Can you work these out from the model? Positions are in its coordinate system, mm. Face numbers are marked on the shaded views. A direction names the side the tool comes from. Round coordinates to 2 decimals unless told otherwise and drop trailing zeros. Order: outer loops, then holes, each group sorted by start corner. A loop starts at its lowest first (then second) coordinate and runs counter-clockwise, first axis right, second up. Notation, with made-up numbers: M -18,16.5 L -9,16.5 A19 cw -9,49.5 Z; hole C 59.25,68 d6. An arc over 180 degrees is marked long. Answer as a JSON object with one key per item and string values. Group by question number.
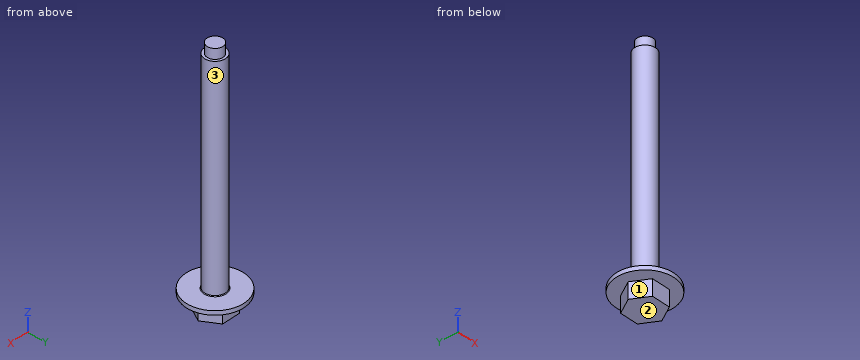
```python
from build123d import *

# Parameters (mm, degrees)
BOSS_EXTRUDE1_DEPTH = 3.175
SKETCH2_R           = 5.715
BOSS_EXTRUDE2_DEPTH = 0.8128
SKETCH3_R           = 2.0701
BOSS_EXTRUDE3_DEPTH = 44.45
FILLET1_R           = 0.127
SKETCH4_OUTSIDE_W   = 23.642
SKETCH4_OUTSIDE_H   = 23.642
SKETCH4_OUTSIDE_R   = 1.5701
CUT_EXTRUDE1_DEPTH  = 1.9812


with BuildPart() as part:
    # Sketch1 → Boss-Extrude1 (new body)
    with BuildSketch(Plane.XY):
        Polygon((3.666174209, 0), (1.833087105, 3.175), (-1.833087105, 3.175), (-3.666174209, 0), (-1.833087105, -3.175), (1.833087105, -3.175), align=None)
    extrude(amount=BOSS_EXTRUDE1_DEPTH)

    # Sketch2 → Boss-Extrude2 (add)
    with BuildSketch(Plane.XY.offset(3.175)):
        Circle(SKETCH2_R)
    extrude(amount=BOSS_EXTRUDE2_DEPTH)

    # Sketch3 → Boss-Extrude3 (add)
    with BuildSketch(Plane.XY.offset(3.9878)):
        Circle(SKETCH3_R)
    extrude(amount=BOSS_EXTRUDE3_DEPTH)

    # Fillet1
    fillet1_edges = [part.edges().sort_by_distance(p)[0] for p in [
        (-2.0701, 0, 3.9878),
    ]]
    fillet(fillet1_edges, radius=FILLET1_R)

    # Sketch4 outside → Cut-Extrude1 (cut)
    with BuildSketch(Plane.XY.offset(48.4378)):
        Rectangle(SKETCH4_OUTSIDE_W, SKETCH4_OUTSIDE_H)
        Circle(SKETCH4_OUTSIDE_R, mode=Mode.SUBTRACT)
    extrude(amount=-CUT_EXTRUDE1_DEPTH, mode=Mode.SUBTRACT)


solid = part.part
```
1) If we section it at D-D on y = 5: Write out the boundary of the cut face in (x, z) (3 decimals), plus the area to 3 significant figures.
2) If we section it at C-C on y = -2.75: Write out the boundary of the cut face in (x, z) (3 decimals).
3) If we section it at B-B on z = 36.5: Write out the boundary of the cut face in (x, y).
4) If we section it at A-A on x = 0: Write out the boundary of the cut face in (y, z) (3 decimals), plus the area to 3 significant figures.
5) I need wall thicknesses on line 1 along Z through (x, y) = (-0.5, -5) (3 decimals); line 2 along Z through (x, y) = (-1.5, -1.25); line 3 along X through (y, z) = (-1, 9.5). Which ranges of each line are inside material? Lowest first, please.
6) For pin 1 (3 mm diameter, centred on x = 1.5, z = 7, fed in from -Y); pin 2 (2.5 mm diameter, centred on x = 0.5, z = 1, fed in from -Y) (3 decimals); pin 3 (1 mm diameter, centred on x = 0.5, z = 1.5, fed in from +Y) (3 decimals), each with a flat end and sliding along its axis, tell me the tip position at first contact or that it passes through.
7) Which directions (+Z, -Z, +X, -X, +Y, -Y) give clear straight access to the entire face, cutting with the end or side of a thin tool? Please do the marked faces 1, 2 and 3.
Findings:
{
 "1": {"outline": "M -2.768,3.175 L 2.768,3.175 L 2.768,3.988 L -2.768,3.988 Z", "area": "4.50 mm^2"},
 "2": {"outline": "M -5.01,3.175 L -2.078,3.175 L -2.078,0 L 2.078,0 L 2.078,3.175 L 5.01,3.175 L 5.01,3.988 L -5.01,3.988 Z"},
 "3": {"outline": "C 0,0 d4.14"},
 "4": {"outline": "M -5.715,3.175 L -3.175,3.175 L -3.175,0 L 3.175,0 L 3.175,3.175 L 5.715,3.175 L 5.715,3.988 L 2.197,3.988 A0.127 cw 2.07,4.115 L 2.07,46.457 L 1.57,46.457 L 1.57,48.438 L -1.57,48.438 L -1.57,46.457 L -2.07,46.457 L -2.07,4.115 A0.127 cw -2.197,3.988 L -5.715,3.988 Z", "area": "212 mm^2"},
 "5": {"line 1": "z = 3.175 to 3.988", "line 2": "z = 0 to 46.46", "line 3": "x = -1.81 to 1.81"},
 "6": {"pin 1": "stops at y = -2.07", "pin 2": "stops at y = -3.175", "pin 3": "stops at y = 3.175"},
 "7": {"face 1": "-Z, -X, -Y", "face 2": "-Z, +X, -X, +Y, -Y", "face 3": "+Z"}
}
